from build123d import *

# Parameters (mm, degrees)
ESQUISSE1_R             = 3.3
ESQUISSE1_R_2           = 2.75
BOSS_EXTRU_1_DEPTH      = 10
ESQUISSE2_R             = 6
ENL_V_MAT_EXTRU_1_DEPTH = 5
ENL_V_MAT_EXTRU_3_DEPTH = 7


with BuildPart() as part:
    # Esquisse1 → Boss.-Extru.1 (new body)
    with BuildSketch(Plane.XY):
        Polygon((6.821863894, 43.038413396), (6.821863894, -36.961586604), (-18.178136106, -36.961586604), (-18.178136106, -11.961586604), (-58.178136106, -11.961586604), (-58.178136106, 18.038413396), (-18.178136106, 18.038413396), (-18.178136106, 43.038413396), align=None)
        with Locations((0.821863894, 26.038413396)):
            Circle(ESQUISSE1_R, mode=Mode.SUBTRACT)
        with Locations((-12.178136106, 26.038413396)):
            Circle(ESQUISSE1_R, mode=Mode.SUBTRACT)
        with Locations((-12.178136106, -19.961586604)):
            Circle(ESQUISSE1_R, mode=Mode.SUBTRACT)
        with Locations((0.821863894, -19.961586604)):
            Circle(ESQUISSE1_R, mode=Mode.SUBTRACT)
        with Locations((-48.178136106, 13.038413396)):
            Circle(ESQUISSE1_R_2, mode=Mode.SUBTRACT)
        with Locations((-28.178136106, 13.038413396)):
            Circle(ESQUISSE1_R_2, mode=Mode.SUBTRACT)
        with Locations((-28.178136106, -6.961586604)):
            Circle(ESQUISSE1_R_2, mode=Mode.SUBTRACT)
        with Locations((-48.178136106, -6.961586604)):
            Circle(ESQUISSE1_R_2, mode=Mode.SUBTRACT)
    extrude(amount=BOSS_EXTRU_1_DEPTH)

    # Esquisse2 → Enlèv. mat.-Extru.1 (cut)
    with BuildSketch(Plane.XY.offset(10)):
        with Locations((-48.178136106, 13.038413396)):
            Circle(ESQUISSE2_R)
        with Locations((-28.178136106, 13.038413396)):
            Circle(ESQUISSE2_R)
        with Locations((-28.178136106, -6.961586604)):
            Circle(ESQUISSE2_R)
        with Locations((-48.178136106, -6.961586604)):
            Circle(ESQUISSE2_R)
    extrude(amount=-ENL_V_MAT_EXTRU_1_DEPTH, mode=Mode.SUBTRACT)

    # Esquisse3 → Enlèv. mat.-Extru.3 (cut)
    with BuildSketch(Plane(origin=(0, 0, 0), x_dir=(-1, 0, 0), z_dir=(0, 0, -1))):
        with BuildLine():
            Line((-0.821863894, 33.038413396), (12.178136106, 33.038413396))
            ThreePointArc((12.178136106, 33.038413396), (19.178136106, 26.038413396), (12.178136106, 19.038413396))
            Line((12.178136106, 19.038413396), (-0.821863894, 19.038413396))
            ThreePointArc((-0.821863894, 19.038413396), (-7.821863894, 26.038413396), (-0.821863894, 33.038413396))
        make_face()
        with BuildLine():
            Line((-0.821863894, -12.961586604), (12.178136106, -12.961586604))
            ThreePointArc((12.178136106, -12.961586604), (19.178136106, -19.961586604), (12.178136106, -26.961586604))
            Line((12.178136106, -26.961586604), (-0.821863894, -26.961586604))
            ThreePointArc((-0.821863894, -26.961586604), (-7.821863894, -19.961586604), (-0.821863894, -12.961586604))
        make_face()
    extrude(amount=-ENL_V_MAT_EXTRU_3_DEPTH, mode=Mode.SUBTRACT)


solid = part.part
Here's how the part is built. I have some questions about the finished solid (model axes, mm). A direction names the side the tool comes from. Give positions to 0.01 mm unless a question says otherwise; leave off trailing zeros. Loops run counter-clockwise (first coordinate to the right, second up) from the corner with the lowest first, then second, coordinate; pieces in that order, holes last. Notation, with made-up numbers: (6.25, 66.25) -> (27.25, 66.25) arc R29 ccw to (27.25, 91.25) -> close; hole circle Ø3 at (0.5, 55.25). An arc over 180 degrees is marked (long way). One line per item, written item: value.
Q1. We'd pull the mould along X, two halves only. Please class faces 1 (the face through (-45.555, 13.864, 2.465)), 2 (the face through (-6, 43.038, 5)): pulls with the +X half, pulls with the -X half, needs draft (parallel to the pull), parting line crosses it, or undercut.
Answers follow:
face 1: undercut
face 2: needs draft
Q2. Suppose I cut it at D-D on x = -36.5. Please give me the cut outline in (y, z), then the cut area to 3 significant figures.
Answers follow:
outline: (-11.96, 0) -> (18.04, 0) -> (18.04, 10) -> (-11.96, 10) -> close
area: 300 mm^2
Q3. Suppose I cut it at B-B on x = -26.5. Please give me the cut outline in (y, z), then the cut area to 3 significant figures.
Answers follow:
outline: (-11.96, 0) -> (-9.14, 0) -> (-9.14, 5) -> (-11.96, 5) -> close; (-4.78, 0) -> (10.86, 0) -> (10.86, 5) -> (7.28, 5) -> (7.28, 10) -> (-1.2, 10) -> (-1.2, 5) -> (-4.78, 5) -> close; (15.22, 0) -> (18.04, 0) -> (18.04, 5) -> (15.22, 5) -> close
area: 149 mm^2
Q4. I'm going to push flat-ended pins straight in: pin 1 Ø3 at (y, z) = (-30.5, 3.5) entering from -X; pin 2 Ø6 at (x, z) = (-43.5, 5) entering from +Y; pin 3 Ø5.5 at (x, y) = (-50, 13.5) entering from +Z; pin 4 Ø6 at (x, y) = (0.82, 26.04) entering from +Z. Where does each tip first touch, or does it pass through?
Answers follow:
pin 1: x = -18.18
pin 2: y = 18.04
pin 3: z = 5
pin 4: through
Q5. Suppose I cut it at C-C on y = 32. Please give me the cut outline in (x, z).
Answers follow:
outline: (-18.18, 0) -> (-15.85, 0) -> (-15.85, 7) -> (4.49, 7) -> (4.49, 0) -> (6.82, 0) -> (6.82, 10) -> (-18.18, 10) -> close
Q6. On a 3-axis mill with a long thin cutter (end or side, diameter ignored), from which of +Z, -Z, +X, -X, +Y, -Y can I reach the whole of each face in a straight line? I mean faces 3 (the face through (0.39, -16.69, 8.48)), 4 (the face through (-47.963, -0.965, 7.535)), 5 (the face through (4.22, -26.08, 3.45)). Say none if no direction works.
Answers follow:
face 3: +Z, -Z
face 4: +Z
face 5: -Z
Q7. Suppose I cut it at A-A on z = 2.75. Please give me the cut outline in (x, y).
Answers follow:
outline: (-58.18, -11.96) -> (-18.18, -11.96) -> (-18.18, -16.36) arc R7 cw to (-12.18, -12.96) -> (0.82, -12.96) arc R7 cw to (6.82, -16.36) -> (6.82, 22.43) arc R7 cw to (0.82, 19.04) -> (-12.18, 19.04) arc R7 cw to (-18.18, 22.43) -> (-18.18, 18.04) -> (-58.18, 18.04) -> close; (-18.18, -36.96) -> (6.82, -36.96) -> (6.82, -23.57) arc R7 cw to (0.82, -26.96) -> (-12.18, -26.96) arc R7 cw to (-18.18, -23.57) -> close; (-18.18, 29.64) arc R7 cw to (-12.18, 33.04) -> (0.82, 33.04) arc R7 cw to (6.82, 29.64) -> (6.82, 43.04) -> (-18.18, 43.04) -> close; hole circle Ø5.5 at (-48.18, -6.96); hole circle Ø5.5 at (-48.18, 13.04); hole circle Ø5.5 at (-28.18, -6.96); hole circle Ø5.5 at (-28.18, 13.04)
Q8. If I drill on line 1 along Y through (x, z) = (1, 5.5); line 2 along X through (y, z) = (13, 8.25); line 3 along Y through (x, z) = (0, 7.75), over which ranges is the centre line in solid material (lowest first)?
Answers follow:
line 1: -36.96 to -26.96, -12.96 to 19.04, 33.04 to 43.04
line 2: -58.18 to -54.18, -42.18 to -34.18, -22.18 to 6.82
line 3: -36.96 to -23.16, -16.77 to 22.84, 29.23 to 43.04
